Source: CAD feature listing. Evaluate the final solid. Frame: model axes, mm. Round coordinates to 2 decimals unless told otherwise and drop trailing zeros. Loops run counter-clockwise (first coordinate to the right, second up) from the corner with the lowest first, then second, coordinate; pieces in that order, holes last. Notation, with made-up numbers: (-40, 33.5) -> (-16, 33.5) arc R15 ccw to (-16, 57.5) -> close; hole circle Ø11 at (72, 47.25). An arc over 180 degrees is marked (long way). Write item = value, one per line.
Autodesk Fusion 360 part; units mm, degrees
sketch "plate-2026-01-10T16_34_53.983Z" plane through (0, 0, 0) normal (0, 0, 1) x (1, 0, 0)
  line L0 (3.025, -21.575) -> (16.025, -21.575)
  line L1 (3.025, -35.575) -> (16.025, -35.575)
  line L2 (2.525, -22.075) -> (2.525, -35.075)
  line L3 (16.525, -22.075) -> (16.525, -35.075)
  arc A0 (3.025, -21.575) -> (2.525, -22.075) centre (3.025, -22.075) ccw
  arc A1 (16.525, -22.075) -> (16.025, -21.575) centre (16.025, -22.075) ccw
  arc A2 (2.525, -35.075) -> (3.025, -35.575) centre (3.025, -35.075) ccw
  arc A3 (16.025, -35.575) -> (16.525, -35.075) centre (16.025, -35.075) ccw
  line L4 (3.025, -40.625) -> (16.025, -40.625)
  line L5 (3.025, -54.625) -> (16.025, -54.625)
  line L6 (2.525, -41.125) -> (2.525, -54.125)
  line L7 (16.525, -41.125) -> (16.525, -54.125)
  arc A4 (3.025, -40.625) -> (2.525, -41.125) centre (3.025, -41.125) ccw
  arc A5 (16.525, -41.125) -> (16.025, -40.625) centre (16.025, -41.125) ccw
  arc A6 (2.525, -54.125) -> (3.025, -54.625) centre (3.025, -54.125) ccw
  arc A7 (16.025, -54.625) -> (16.525, -54.125) centre (16.025, -54.125) ccw
  line L8 (3.025, -59.675) -> (16.025, -59.675)
  line L9 (3.025, -73.675) -> (16.025, -73.675)
  line L10 (2.525, -60.175) -> (2.525, -73.175)
  line L11 (16.525, -60.175) -> (16.525, -73.175)
  arc A8 (3.025, -59.675) -> (2.525, -60.175) centre (3.025, -60.175) ccw
  arc A9 (16.525, -60.175) -> (16.025, -59.675) centre (16.025, -60.175) ccw
  arc A10 (2.525, -73.175) -> (3.025, -73.675) centre (3.025, -73.175) ccw
  arc A11 (16.025, -73.675) -> (16.525, -73.175) centre (16.025, -73.175) ccw
  line L12 (3.025, -78.725) -> (16.025, -78.725)
  line L13 (3.025, -92.725) -> (16.025, -92.725)
  line L14 (2.525, -79.225) -> (2.525, -92.225)
  line L15 (16.525, -79.225) -> (16.525, -92.225)
  arc A12 (3.025, -78.725) -> (2.525, -79.225) centre (3.025, -79.225) ccw
  arc A13 (16.525, -79.225) -> (16.025, -78.725) centre (16.025, -79.225) ccw
  arc A14 (2.525, -92.225) -> (3.025, -92.725) centre (3.025, -92.225) ccw
  arc A15 (16.025, -92.725) -> (16.525, -92.225) centre (16.025, -92.225) ccw
  line L16 (-12.565, 4.91) -> (77.435, 4.91)
  line L17 (77.435, 4.91) -> (77.435, -106.09)
  line L18 (77.435, -106.09) -> (-12.565, -106.09)
  line L19 (-12.565, -106.09) -> (-12.565, 4.91)
  line L20 (38.056, 4.91) -> (56.556, 4.91)
  line L21 (56.556, 4.91) -> (56.556, -26.09)
  line L22 (56.556, -26.09) -> (38.056, -26.09)
  line L23 (38.056, -26.09) -> (38.056, 4.91)
  circle A16 centre (-7.565, -101.09) radius 1.7
  circle A17 centre (72.435, -101.09) radius 1.7
  circle A18 centre (72.435, -0.09) radius 1.7
  circle A19 centre (-7.565, -0.09) radius 1.7
  dimension "d1" = 111
  dimension "d2" = 90
  dimension "d3" = 15.09
  dimension "d4" = 13.365
  dimension "d5" = 18.5
  dimension "d6" = 31
  dimension "d7" = 50.621
  dimension "d8" = 3.4
  dimension "d9" = 5
  dimension "d10" = 5
  dimension "d11" = 3.4
  dimension "d12" = 5
  dimension "d13" = 5
  dimension "d14" = 3.4
  dimension "d15" = 5
  dimension "d16" = 5
  dimension "d17" = 3.4
  dimension "d18" = 5
  dimension "d19" = 5
sketch "Sketch2" plane through (0, 0, 0) normal (0, 0, 1) x (1, 0, 0)
sketch "Sketch3" plane through (0, 0, 0) normal (0, 0, 1) x (1, 0, 0)
extrude "Extrude1" add sketch "plate-2026-01-10T16_34_53.983Z" along normal blind 1.5 contours L16 L17 L18 L19 L21 L22 L23
fillet "Fillet1" radius 5 1 edges at (77.435, -106.09, 0.75)
fillet "Fillet2" radius 5 1 edges at (77.435, 4.91, 0.75)
fillet "Fillet3" radius 5 1 edges at (-12.565, 4.91, 0.75)
fillet "Fillet4" radius 5 1 edges at (-12.565, -106.09, 0.75)
1. Mould query, pull axis X, two halves, no side actions, for faces 1 (the face through (32, -50, 0)), 2 (the face through (-11.061, 3.484, 0.76)), 3 (the face through (76.009, 3.406, 0.76)), 4 (the face through (74.056, -101.601, 0.74)). Classes: released by +X, released by -X, zero draft, split by the parting line, or undercut.
Evaluation:
face_1 = zero draft
face_2 = released by -X
face_3 = released by +X
face_4 = undercut
2. Section query D-D (y = -9.5). Return the cut outline in (x, z) (3 decimals), then the cut area to 3 significant figures.
Evaluation:
outline = (-12.565, 0) -> (38.056, 0) -> (38.056, 1.5) -> (-12.565, 1.5) -> close; (56.556, 0) -> (77.435, 0) -> (77.435, 1.5) -> (56.556, 1.5) -> close
area = 107 mm²
3. Contact query for a flat-ended pin moving along its axis: pin 1 Ø2 at (x, y) = (72.435, -101.09) entering from +Z. Output: stop coordinate, or through.
Evaluation:
pin_1 = through
4. Section query A-A (y = -44). Return the cut outline in (x, z) (3 decimals), then the cut area to 3 significant figures.
Evaluation:
outline = (-12.565, 0) -> (2.525, 0) -> (2.525, 1.5) -> (-12.565, 1.5) -> close; (16.525, 0) -> (77.435, 0) -> (77.435, 1.5) -> (16.525, 1.5) -> close
area = 114 mm²
5. Section query B-B (x = 6). Return the cut outline in (y, z) (3 decimals), then the cut area to 3 significant figures.
Evaluation:
outline = (-106.09, 0) -> (-92.725, 0) -> (-92.725, 1.5) -> (-106.09, 1.5) -> close; (-78.725, 0) -> (-73.675, 0) -> (-73.675, 1.5) -> (-78.725, 1.5) -> close; (-59.675, 0) -> (-54.625, 0) -> (-54.625, 1.5) -> (-59.675, 1.5) -> close; (-40.625, 0) -> (-35.575, 0) -> (-35.575, 1.5) -> (-40.625, 1.5) -> close; (-21.575, 0) -> (4.91, 0) -> (4.91, 1.5) -> (-21.575, 1.5) -> close
area = 82.5 mm²
6. Line query: probe 1 along X at (y, z) = (-101.09, 0.9) (3 decimals); probe 2 along X at (y, z) = (-24.5, 1.3) (3 decimals); probe 3 along Y at (x, z) = (5, 1.2) (3 decimals). Output: solid intervals per line, ascending. Write a range as from..to.
Evaluation:
probe_1 = -12.565..-9.265, -5.865..70.735, 74.135..77.435
probe_2 = -12.565..2.525, 16.525..38.056, 56.556..77.435
probe_3 = -106.09..-92.725, -78.725..-73.675, -59.675..-54.625, -40.625..-35.575, -21.575..4.91
7. Section query C-C (z = 0.3). Give the number of separate pieces and of enclosed holes in the cut face, then the cut area to 3 significant figures.
Evaluation:
separate_pieces = 1
enclosed_holes = 8
area = 8,580 mm²
